Model file for the job. Use its own axes, mm. A direction names the side the tool comes from. Round coordinates to 2 decimals unless told otherwise and drop trailing zeros. Loops run counter-clockwise (first coordinate to the right, second up) from the corner with the lowest first, then second, coordinate; pieces in that order, holes last. Notation, with made-up numbers: (-9, -3) -> (50, -3) arc R22 cw to (50, 23) -> close; hole circle Ø6 at (82, 32). An arc over 180 degrees is marked (long way). Use a Markdown table: item, result. Add a question column.
```python
from build123d import *

# Parameters (mm, degrees)
CROQUIS1_R              = 1.75
SALIENTE_EXTRUIR1_DEPTH = 5.5
SALIENTE_EXTRUIR2_DEPTH = 11


with BuildPart() as part:
    # Croquis1 → Saliente-Extruir1 (new, symmetric)
    with BuildSketch(Plane(origin=(0, 0, 0), x_dir=(1, 0, 0), z_dir=(0, 1, 0))):
        with BuildLine():
            Line((-6.9961079, -3.195655599), (-105.176277572, 171.04743403))
            Line((-105.176277572, 171.04743403), (-93.698060534, 171.04743403))
            Line((-93.698060534, 171.04743403), (-11.69265741, 25.510154411))
            Line((-11.69265741, 25.510154411), (-5.393659345, 25.510154411))
            ThreePointArc((-5.393659345, 25.510154411), (-2.426146714, 23.865920772), (-2.246796422, 20.478079431))
            Line((-2.246796422, 20.478079431), (-5.310946382, 14.184353585))
            Line((-5.310946382, 14.184353585), (1.716046582, 1.713352885))
            ThreePointArc((1.716046582, 1.713352885), (-0.185526417, -5.097228597), (-6.9961079, -3.195655599))
        make_face()
        with Locations(Location((-5.393659345, 22.010154411, 0), (0, 0, 270))):
            Circle(CROQUIS1_R, mode=Mode.SUBTRACT)
        with Locations(Location((-6.567237446, 6.228572228, 0), (0, 0, 270))):
            Circle(CROQUIS1_R, mode=Mode.SUBTRACT)
    extrude(amount=SALIENTE_EXTRUIR1_DEPTH, both=True)

    # Croquis3 → Saliente-Extruir2 (add)
    with BuildSketch(Plane(origin=(0, 5.5, 0), x_dir=(1, 0, 0), z_dir=(0, 1, 0))):
        with BuildLine():
            Line((-12.150815645, -2.195736734), (-5.150815645, -5.065033727))
            ThreePointArc((-5.150815645, -5.065033727), (-6.19841412, -4.253687071), (-6.9961079, -3.195655599))
            Line((-6.9961079, -3.195655599), (-16.8311389, 14.258848643))
            Line((-16.8311389, 14.258848643), (-16.837857523, 9.178094271))
            Line((-16.837857523, 9.178094271), (-12.150815645, -2.195736734))
        make_face()
    extrude(amount=-SALIENTE_EXTRUIR2_DEPTH)


solid = part.part
```
1) Wall check: probe 1 along X at (y, z) = (-3.5, -82); probe 2 along X at (y, z) = (3.25, -138); probe 3 along Z at (x, y) = (-83, -0.5). Give the ranges that are in metal, low to high. Write a range as from..to.
2) Cut at B-B on z = -76.5. Write the cut outline in (x, y), and give its area (3 significant figures).
3) Cut at A-A on y = -1.5. Write the cut outline in (x, z), and give its area (3 significant figures).
4) Pull direction Z, two halves, no side cores. Call faces 1 (the face through (-3.757, 0.077, -17.375)), 2 (the face through (-14.527, 0.077, -3.571)), 3 (the face through (-6.06, -0.08, -20.39)), 4 (the face through (-48, -5.5, -77)): +Z half, -Z half, draft (parallel to the pull), parting line (faces both ways), or undercut.
5) Cut at C-C on x = -31. Write the cut outline in (y, z), and give its area (3 significant figures).
6) Pin check, flat tips, straight feed: pin 1 Ø5 at (x, y) = (-7.5, 2.5) entering from -Z; pin 2 Ø6 at (x, y) = (-70, -3) entering from -Z; pin 3 Ø1.5 at (x, y) = (-12, -1) entering from -Z. Stop position of each tip, or through.
7) Tool access for faces 5 (the face through (-1.85, 0.08, -8.04)), 6 (the face through (-8.7, 0.08, 3.61)), 7 (the face through (-9, 0, -25.51)): list every direction of +Z, -Z, +X, -X, +Y, -Y with a clear straight run to the whole face (end or side of a thin tool).
Established:
| question | item | result |
|---|---|---|
| 1 | probe 1 | x = -55..-43.52 |
| 1 | probe 2 | x = -86.56..-75.08 |
| 1 | probe 3 | z = -152.06..-131.69 |
| 2 | outline | (-51.9, -5.5) -> (-40.42, -5.5) -> (-40.42, 5.5) -> (-51.9, 5.5) -> close |
| 2 | area | 126 mm^2 |
| 3 | outline | (-105.18, -171.05) -> (-93.7, -171.05) -> (-11.69, -25.51) -> (-5.39, -25.51) arc R3.5 ccw to (-2.25, -20.48) -> (-5.31, -14.18) -> (1.72, -1.71) arc R5 ccw to (-5.15, 5.07) -> (-12.15, 2.2) -> (-16.84, -9.18) -> (-16.83, -14.26) -> close; hole circle Ø3.5 at (-6.57, -6.23); hole circle Ø3.5 at (-5.39, -22.01) |
| 3 | area | 2,110 mm^2 |
| 4 | face 1 | undercut |
| 4 | face 2 | +Z half |
| 4 | face 3 | undercut |
| 4 | face 4 | draft |
| 5 | outline | (-5.5, -59.78) -> (5.5, -59.78) -> (5.5, -39.4) -> (-5.5, -39.4) -> close |
| 5 | area | 224 mm^2 |
| 6 | pin 1 | stops at z = -25.51 |
| 6 | pin 2 | stops at z = -134.31 |
| 6 | pin 3 | stops at z = -27.39 |
| 7 | face 5 | +X, +Y, -Y |
| 7 | face 6 | +Z, -X, +Y, -Y |
| 7 | face 7 | -Z, +X, +Y, -Y |
